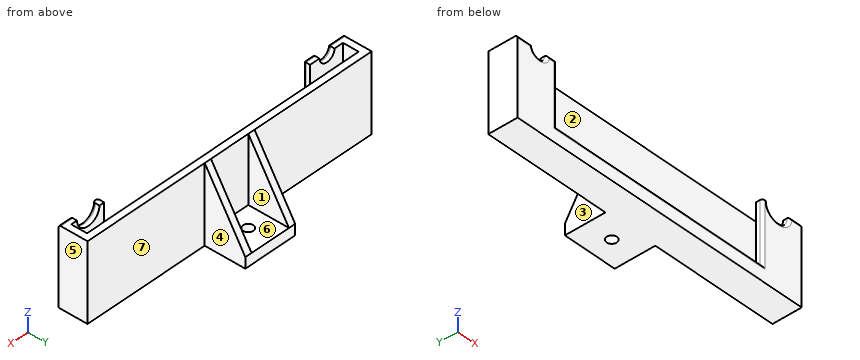
```python
from build123d import *

# Parameters (mm, degrees)
F0_W          = 144.78
F0_H          = 13.716
F1_DEPTH      = 36.195
F2_W          = 138.43
F2_H          = 7.366
F3_DEPTH      = 33.02
F4_W          = 104.902
F4_H          = 28.956
F5_DEPTH      = 3.175
F6_W          = 25.4
F6_H          = 19.05
F7_DEPTH      = 36.195
F8_W          = 19.05
F8_H          = 19.05
F9_DEPTH      = 31.115
F11_DEPTH     = 25.4
F12_R         = 2.38125
F13_DEPTH     = 25.4
F14_R         = 9.525
F15_T1_DEPTH  = 104.902
F15_T3_DEPTH  = 13.843
F15_T5_DEPTH  = 11.176
F15_T7_DEPTH  = 12.446
F15_T9_DEPTH  = 32.131
F15_T12_ANGLE = 243.7643577336
F15_T14_ANGLE = 275.6465366004
F15_T19_DEPTH = 108.077
F15_T23_DEPTH = 32.131
F15_T30_DEPTH = 32.131
F15_T34_DEPTH = 108.077


# Not quite as in the source:
# - a fillet or chamfer that OpenCascade refuses, or shapes differently, is made with other operations: its cross-section is extruded or revolved along the edge and cut away or added


with BuildPart() as f1:
    # F0 (on Top) → F1 (new body)
    with BuildSketch(Plane.XY):
        with Locations((72.39, 6.858)):
            Rectangle(F0_W, F0_H)
    extrude(amount=F1_DEPTH)

    # F2 (on face) → F3 (cut)
    with BuildSketch(Plane.XY.offset(36.195)):
        with Locations((72.39, 6.858)):
            Rectangle(F2_W, F2_H)
    extrude(amount=-F3_DEPTH, mode=Mode.SUBTRACT)

    # F4 (on face) → F5 (cut)
    with BuildSketch(Plane.XZ):
        with BuildLine():
            ThreePointArc((7.493, 36.195), (11.303, 32.385), (15.113, 36.195))
            Line((15.113, 36.195), (7.493, 36.195))
        make_face()
        with Locations((72.39, 21.717)):
            Rectangle(F4_W, F4_H)
        with BuildLine():
            Line((138.684, 36.195), (127.254, 36.195))
            ThreePointArc((127.254, 36.195), (132.969, 30.48), (138.684, 36.195))
        make_face()
    extrude(amount=-F5_DEPTH, mode=Mode.SUBTRACT)

    # F6 (on Top) → F7 (join)
    with BuildSketch(Plane.XY):
        with Locations((72.39, 23.241)):
            Rectangle(F6_W, F6_H)
    extrude(amount=F7_DEPTH)

    # F8 (on face) → F9 (cut)
    with BuildSketch(Plane.XY.offset(36.195)):
        with Locations((72.39, 23.241)):
            Rectangle(F8_W, F8_H)
    extrude(amount=-F9_DEPTH, mode=Mode.SUBTRACT)

    # F10 (on face) → F11 (cut)
    with BuildSketch(Plane.YZ.offset(85.09)):
        Polygon((32.766, 36.195), (13.716, 36.195), (32.766, 5.08), align=None)
    extrude(amount=-F11_DEPTH, mode=Mode.SUBTRACT)

    # F12 (on face) → F13 (cut)
    with BuildSketch(Plane(origin=(0, 0, 0), x_dir=(1, 0, 0), z_dir=(0, 0, -1))):
        with Locations((72.39, -22.44725)):
            Circle(F12_R)
    extrude(amount=-F13_DEPTH, mode=Mode.SUBTRACT)

    # F14
    f14_edges = [f1.edges().sort_by_distance(p)[0] for p in [
        (141.605, 6.858, 3.175),
        (3.175, 6.858, 3.175),
    ]]
    fillet(f14_edges, radius=F14_R)

    # F15: fillet of radius 1.27 on 9 edges, made by hand

    # F15_s2 → F15_t1 (cut)
    with BuildSketch(Plane.YZ.offset(19.939)):
        with BuildLine():
            ThreePointArc((1.27, 7.239), (0.3719743879, 6.8670256121), (0, 5.969))
            Line((0, 5.969), (0, 7.239))
            Line((0, 7.239), (1.27, 7.239))
        make_face()
    extrude(amount=F15_T1_DEPTH, mode=Mode.SUBTRACT)

    # F15_s4 → F15_t3 (cut)
    with BuildSketch(Plane.YZ.offset(-3.175)):
        with BuildLine():
            ThreePointArc((1.27, 36.195), (0.3719743879, 35.8230256121), (0, 34.925))
            Line((0, 34.925), (0, 36.195))
            Line((0, 36.195), (1.27, 36.195))
        make_face()
    extrude(amount=F15_T3_DEPTH, mode=Mode.SUBTRACT)

    # F15_s6 → F15_t5 (cut)
    with BuildSketch(Plane.YZ.offset(11.938)):
        with BuildLine():
            ThreePointArc((1.27, 36.195), (0.3719743879, 35.8230256121), (0, 34.925))
            Line((0, 34.925), (0, 36.195))
            Line((0, 36.195), (1.27, 36.195))
        make_face()
    extrude(amount=F15_T5_DEPTH, mode=Mode.SUBTRACT)

    # F15_s8 → F15_t7 (cut)
    with BuildSketch(Plane.YZ.offset(135.509)):
        with BuildLine():
            ThreePointArc((1.27, 36.195), (0.3719743879, 35.8230256121), (0, 34.925))
            Line((0, 34.925), (0, 36.195))
            Line((0, 36.195), (1.27, 36.195))
        make_face()
    extrude(amount=F15_T7_DEPTH, mode=Mode.SUBTRACT)

    # F15_s10 → F15_t9 (cut)
    with BuildSketch(Plane.XY.offset(7.239)):
        with BuildLine():
            ThreePointArc((19.939, 1.27), (19.5670256121, 0.3719743879), (18.669, 0))
            Line((18.669, 0), (19.939, 0))
            Line((19.939, 0), (19.939, 1.27))
        make_face()
        with BuildLine():
            ThreePointArc((124.841, 1.27), (125.2129743879, 0.3719743879), (126.111, 0))
            Line((126.111, 0), (124.841, 0))
            Line((124.841, 0), (124.841, 1.27))
        make_face()
    extrude(amount=F15_T9_DEPTH, mode=Mode.SUBTRACT)

    # F15_s11 → F15_t12 (revolve, cut)
    with BuildSketch(Plane(origin=(53.3272604269, 0, 85.7332545483), x_dir=(0, 1, 0), z_dir=(0.5281742472, 0, 0.8491360107))):
        with BuildLine():
            ThreePointArc((1.27, -88.0764993266), (0.3719743879, -87.7045249387), (0, -86.8064993266))
            Line((0, -86.8064993266), (0, -88.0764993266))
            Line((0, -88.0764993266), (1.27, -88.0764993266))
        make_face()
    revolve(axis=Axis((132.969, 0, 36.195), (0, -1, 0)), revolution_arc=F15_T12_ANGLE, mode=Mode.SUBTRACT)

    # F15_s13 → F15_t14 (revolve, cut)
    with BuildSketch(Plane(origin=(24.217245462, 0, 21.9409429798), x_dir=(0, 1, 0), z_dir=(0.7410773266, 0, 0.6714196869))):
        with BuildLine():
            ThreePointArc((1.27, 23.0442371148), (0.3719743879, 23.4162115027), (0, 24.3142371148))
            Line((0, 24.3142371148), (0, 23.0442371148))
            Line((0, 23.0442371148), (1.27, 23.0442371148))
        make_face()
    revolve(axis=Axis((11.303, 0, 36.195), (0, -1, 0)), revolution_arc=F15_T14_ANGLE, mode=Mode.SUBTRACT)


with BuildPart() as f15_tool17:
    # F15_s18 → F15_t19 (new body)
    with BuildSketch(Plane.YZ.offset(16.764)):
        with BuildLine():
            ThreePointArc((1.27, 7.239), (0.3719743879, 6.8670256121), (0, 5.969))
            Line((0, 5.969), (0, 7.239))
            Line((0, 7.239), (1.27, 7.239))
        make_face()
    extrude(amount=F15_T19_DEPTH)

    split(bisect_by=Plane.YZ.offset(19.939), keep=Keep.BOTTOM)


with BuildPart() as f15_tool21:
    # F15_s22 → F15_t23 (new body)
    with BuildSketch(Plane.XY.offset(36.195)):
        with BuildLine():
            ThreePointArc((19.939, 1.27), (19.5670256121, 0.3719743879), (18.669, 0))
            Line((18.669, 0), (19.939, 0))
            Line((19.939, 0), (19.939, 1.27))
        make_face()
    extrude(amount=-F15_T23_DEPTH)

    split(bisect_by=Plane.XY.offset(7.239), keep=Keep.BOTTOM)


with BuildPart() as f15_tool17_1:
    add(f15_tool17.part)

    # F15_t25: intersect F15_tool21
    add(f15_tool21.part, mode=Mode.INTERSECT)


with BuildPart() as f1_1:
    add(f1.part)

    # F15_t15: cut F15_tool17
    add(f15_tool17_1.part, mode=Mode.SUBTRACT)


with BuildPart() as f15_tool28:
    # F15_s29 → F15_t30 (new body)
    with BuildSketch(Plane.XY.offset(4.064)):
        with BuildLine():
            ThreePointArc((124.841, 1.27), (125.2129743879, 0.3719743879), (126.111, 0))
            Line((126.111, 0), (124.841, 0))
            Line((124.841, 0), (124.841, 1.27))
        make_face()
    extrude(amount=F15_T30_DEPTH)

    split(bisect_by=Plane.XY.offset(7.239), keep=Keep.BOTTOM)


with BuildPart() as f15_tool32:
    # F15_s33 → F15_t34 (new body)
    with BuildSketch(Plane.YZ.offset(19.939)):
        with BuildLine():
            ThreePointArc((1.27, 7.239), (0.3719743879, 6.8670256121), (0, 5.969))
            Line((0, 5.969), (0, 7.239))
            Line((0, 7.239), (1.27, 7.239))
        make_face()
    extrude(amount=F15_T34_DEPTH)

    split(bisect_by=Plane.YZ.offset(124.841), keep=Keep.TOP)


with BuildPart() as f15_tool28_1:
    add(f15_tool28.part)

    # F15_t36: intersect F15_tool32
    add(f15_tool32.part, mode=Mode.INTERSECT)


with BuildPart() as f1_2:
    add(f1_1.part)

    # F15_t26: cut F15_tool28
    add(f15_tool28_1.part, mode=Mode.SUBTRACT)


solid = f1_2.part
```
Geometry: final body of the model. Coordinates: model frame, mm. Face numbers are marked on the shaded views. A direction names the side the tool comes from. Round coordinates to 2 decimals unless told otherwise and drop trailing zeros. Loops run counter-clockwise (first coordinate to the right, second up) from the corner with the lowest first, then second, coordinate; pieces in that order, holes last.
Item 1: Section A-A, the plane x = 72.39. Output: boundary loops of the cut face in (y, z) (1 decimal), plus the area to 3 significant figures.
Checked values:
outline: (0, 0) - (20.1, 0) - (20.1, 5.1) - (13.7, 5.1) - (13.7, 36.2) - (10.5, 36.2) - (10.5, 3.2) - (3.2, 3.2) - (3.2, 7.2) - (1.3, 7.2) arc R1.3 ccw to (0, 6) - close; (24.8, 0) - (32.8, 0) - (32.8, 5.1) - (24.8, 5.1) - close
area: 234 mm2
Item 2: Mould query, pull axis X, two halves, no side actions, for the marked faces 5, 6 and 7. Classes: released by +X, released by -X, zero draft, split by the parting line, or undercut.
Checked values:
face 5: released by +X
face 6: undercut
face 7: zero draft
Item 3: Line query: L1, parallel to X at y = 17.5, z = 24 (3 decimals); L2, parallel to Y at x = 101, z = 5 (3 decimals); L3, parallel to X at y = 8, z = 22 (3 decimals). Output: solid intervals per line, ascending.
Checked values:
L1: x = 59.69 to 62.865, 81.915 to 85.09
L2: y = 0 to 3.175, 10.541 to 13.716
L3: x = 0 to 3.175, 141.605 to 144.78
Item 4: Contact query for flat-ended pins moving along their axis: P1, Ø16.5, axis at x = 96, z = 15.5, coming from the +Y side; P2, Ø10, axis at x = 121, z = 14.5, coming from the -Y side; P3, Ø10, axis at x = 61, z = 20.5, coming from the -Y side; P4, Ø3, axis at x = 88, y = 20, coming from the -Z side. Output: stop coordinate, or through.
Checked values:
P1: stops at y = 13.72
P2: stops at y = 0
P3: stops at y = 10.54
P4: passes through
Item 5: Section C-C, the plane x = 30.5. Output: boundary loops of the cut face in (y, z) (3 decimals), plus the area to 3 significant figures.
Checked values:
outline: (0, 0) - (13.716, 0) - (13.716, 36.195) - (10.541, 36.195) - (10.541, 3.175) - (3.175, 3.175) - (3.175, 7.239) - (1.27, 7.239) arc R1.27 ccw to (0, 5.969) - close
area: 161 mm2
Item 6: Reachability of the marked faces 1, 2, 3 and 4 from +Z, -Z, +X, -X, +Y, -Y: full face, straight path, thin tool, end or side. Return the list, or none.
Checked values:
face 1: +Z, +Y
face 2: +Z
face 3: +Z, -Z, -X, +Y
face 4: +Z, -Z, +X, +Y
Item 7: Section D-D, the plane z = 15. Output: boundary loops of the cut face in (x, y) (3 decimals), plus the area to 3 significant figures.
Checked values:
outline: (0, 0) - (18.669, 0) arc R1.27 ccw to (19.939, 1.27) - (19.939, 3.175) - (3.175, 3.175) - (3.175, 10.541) - (141.605, 10.541) - (141.605, 3.175) - (124.841, 3.175) - (124.841, 1.27) arc R1.27 ccw to (126.111, 0) - (144.78, 0) - (144.78, 13.716) - (85.09, 13.716) - (85.09, 26.693) - (81.915, 26.693) - (81.915, 13.716) - (62.865, 13.716) - (62.865, 26.693) - (59.69, 26.693) - (59.69, 13.716) - (0, 13.716) - close
area: 715 mm2
Item 8: Section B-B, the plane y = 9. Output: boundary loops of the cut face in (x, z) (3 decimals).
Checked values:
outline: (0, 0) - (144.78, 0) - (144.78, 36.195) - (141.605, 36.195) - (141.605, 12.7) arc R9.525 cw to (132.08, 3.175) - (12.7, 3.175) arc R9.525 cw to (3.175, 12.7) - (3.175, 36.195) - (0, 36.195) - close
